from build123d import *

# Parameters (mm, degrees)
BOSS_EXTRUDE1_DEPTH = 8
TAPPED_HOLE1_D      = 14.5


with BuildPart() as part:
    # Sketch1 → Boss-Extrude1 (new body)
    with BuildSketch(Plane(origin=(0, 0, 0), x_dir=(0, 0, -1), z_dir=(1, 0, 0))):
        Polygon((13.856406461, 0), (6.92820323, 12), (-6.92820323, 12), (-13.856406461, 0), (-6.92820323, -12), (6.92820323, -12), align=None)
    extrude(amount=BOSS_EXTRUDE1_DEPTH)

    # Tapped Hole1 (through all)
    with Locations(Plane.ZY):
        with Locations((0, 0)):
            Hole(TAPPED_HOLE1_D / 2)

    # Sketch6 → Cut-Revolve1 (revolve, cut)
    with BuildSketch(Plane(origin=(0, 0, 0), x_dir=(1, 0, 0), z_dir=(0, 1, 0))):
        Polygon((0, 12), (1.07179677, 13.856406461), (0, 13.856406461), align=None)
    cut_revolve1 = revolve(axis=Axis((0, 0, 0), (1, 0, 0)), mode=Mode.SUBTRACT)

    # Mirror1: Cut-Revolve1 across plane
    add(cut_revolve1.mirror(Plane.ZY.offset(-4)), mode=Mode.SUBTRACT)


solid = part.part
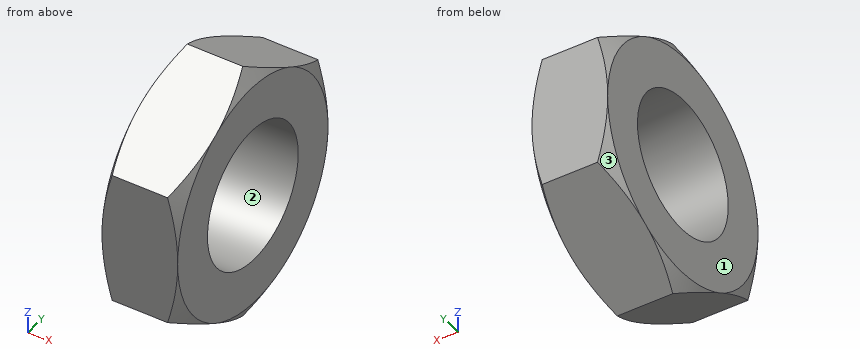
Model file for the job. Use its own axes, mm. Face numbers are marked on the shaded views. Round coordinates to 2 decimals unless told otherwise and drop trailing zeros. Loops run counter-clockwise (first coordinate to the right, second up) from the corner with the lowest first, then second, coordinate; pieces in that order, holes last.
1. Band-saw the part on A-A, the plane x = 4.25. List the corners of the cut face in (y, z).
Check values:
outline: (-12, -6.93) - (0, -13.86) - (12, -6.93) - (12, 6.93) - (0, 13.86) - (-12, 6.93) - close; hole circle Ø14.5 at (0, 0)
2. Drop a flat-ended pin along its axis: P1, Ø1.5, axis at y = -7.5, z = 10.5, coming from the -X side. Give the stop position or say it passes through.
Check values:
P1: passes through
3. Wall check: probe 1 along Z at (x, y) = (2.75, -3); probe 2 along Y at (x, z) = (7, -5.75); probe 3 along Y at (x, z) = (5, 4). Give the ranges that are in metal, low to high.
Check values:
probe 1: z = -12.12 to -6.6, 6.6 to 12.12
probe 2: y = -12 to -4.42, 4.42 to 12
probe 3: y = -12 to -6.05, 6.05 to 12
4. Mould opens along Y. For the marked faces 1, 2 and 3 say: +Y half, -Y half, draft (parallel to the pull), parting line (faces both ways), or undercut.
Check values:
face 1: draft
face 2: undercut
face 3: +Y half
